Work out the finished part from the listing and answer in its coordinate system (mm). A direction names the side the tool comes from. Round coordinates to 2 decimals unless told otherwise and drop trailing zeros. Order: outer loops, then holes, each group sorted by start corner. A loop starts at its lowest first (then second) coordinate and runs counter-clockwise, first axis right, second up. Notation, with made-up numbers: M 54,-30 L 67,-30 A12 cw 67,-17 Z; hole C 71.5,4.5 d5. An arc over 180 degrees is marked long. Answer as a JSON object with one key per item and string values. Group by question number.
from build123d import *

# Parameters (mm, degrees)
F0_W     = 406.4
F0_H     = 304.8
F1_DEPTH = 2.54
F2_W     = 7.62
F2_H     = 7.62
F3_DEPTH = 88.9
F4_W     = 203.2
F4_H     = 203.2
F5_DEPTH = 165.1
F7_DEPTH = 203.2
F8_W     = 7.62
F8_H     = 297.18
F9_DEPTH = 7.62


with BuildPart() as f1:
    # F0 (on Top) → F1 (new body)
    with BuildSketch(Plane.XY):
        with Locations((-190.104838, 115.129152)):
            Rectangle(F0_W, F0_H)
    extrude(amount=F1_DEPTH)

    # F2 (on face) → F3 (join)
    with BuildSketch(Plane.XY.offset(2.54)):
        with Locations((-389.494838, -33.460848)):
            Rectangle(F2_W, F2_H)
        with Locations((9.285162, -33.460848)):
            Rectangle(F2_W, F2_H)
        with Locations((9.285162, 263.719152)):
            Rectangle(F2_W, F2_H)
    extrude(amount=F3_DEPTH)

    # F4 (on face) → F5 (join)
    with BuildSketch(Plane.XY.offset(2.54)):
        with Locations((-291.704838, 165.929152)):
            Rectangle(F4_W, F4_H)
    extrude(amount=F5_DEPTH)

    # F6 (on face) → F7 (join)
    with BuildSketch(Plane.XZ.offset(-64.329152)):
        Polygon((-291.704838, 231.14), (-393.304838, 167.64), (-291.704838, 167.64), align=None)
        Polygon((-291.704838, 231.14), (-291.704838, 167.64), (-190.104838, 167.64), align=None)
    extrude(amount=-F7_DEPTH)

    # F8 (on face) → F9 (join)
    with BuildSketch(Plane.XY.offset(91.44)):
        Polygon((-393.304838, -37.270848), (13.095162, -37.270848), (13.095162, -29.650848), (5.475162, -29.650848), (-393.304838, -29.650848), align=None)
        with Locations((9.285162, 118.939152)):
            Rectangle(F8_W, F8_H)
    extrude(amount=F9_DEPTH)


solid = f1.part
Item 1: Find section C-C (z = 83.5). Give the vertices of the cut face in (x, y).
Item 2: Find section D-D (y = 8). Give the vertices of the cut face in (x, z).
Item 3: Consider L1, parallel to X at y = 93.5, z = 92.5; L2, parallel to Y at x = -272, z = 96; L3, parallel to X at y = 130, z = 14. Determine where each line is inside the solid, lowest interval first.
Item 4: The mould has two halves that part along Y. Classify faces 4 (the flat face through (-341.794, 164.507, 199.834)), 5 (the flat face through (-251, -37.271, 93)), 6 (the flat face through (-283, 267.529, 88)), 7 (the flat face through (-193, -29.651, 93)): +Y half, -Y half, draft (parallel to the pull), parting line (faces both ways), or undercut.
Item 5: Each of these flat-tipped pins is pushed along its axis until it touches: pin 1 (5 mm diameter, centred on y = 143, z = 169, fed in from +X); pin 2 (4 mm diameter, centred on x = -323.5, z = 106.5, fed in from -Y); pin 3 (3 mm diameter, centred on x = -216, y = 4, fed in from +Z). Where does it stop, or does it pass through?
Item 6: Find section B-B (x = -99). Give the vertices of the cut face in (y, z).
Item 7: Find section A-A (y = 200.5). Give the vertices of the cut face in (x, z), and give its area (3 significant figures).
Item 8: A tool of negligible diameter and unlimited length cuts with its end or side. For faces 1 (the flat face through (-293, 64.329, 93)), 2 (the flat face through (-193, 117, 0)), 3 (the flat face through (5.475, 162, 93)), from which of +Z, -Z, +X, -X, +Y, -Y can it reach the whole face along a straight path? Write none if from no direction.
Responses:
{
 "1": {"outline": "M -393.3,-37.27 L -385.68,-37.27 L -385.68,-29.65 L -393.3,-29.65 Z; M -393.3,64.33 L -190.1,64.33 L -190.1,267.53 L -393.3,267.53 Z; M 5.48,-37.27 L 13.1,-37.27 L 13.1,-29.65 L 5.48,-29.65 Z; M 5.48,259.91 L 13.1,259.91 L 13.1,267.53 L 5.48,267.53 Z"},
 "2": {"outline": "M -393.3,0 L 13.1,0 L 13.1,2.54 L -393.3,2.54 Z; M 5.48,91.44 L 13.1,91.44 L 13.1,99.06 L 5.48,99.06 Z"},
 "3": {"L1": "x = -393.3 to -190.1, 5.48 to 13.1", "L2": "y = -37.27 to -29.65, 64.33 to 267.53", "L3": "x = -393.3 to -190.1"},
 "4": {"face 4": "draft", "face 5": "-Y half", "face 6": "+Y half", "face 7": "undercut"},
 "5": {"pin 1": "stops at x = -190.1", "pin 2": "stops at y = 64.33", "pin 3": "stops at z = 2.54"},
 "6": {"outline": "M -37.27,0 L 267.53,0 L 267.53,2.54 L -37.27,2.54 Z; M -37.27,91.44 L -29.65,91.44 L -29.65,99.06 L -37.27,99.06 Z"},
 "7": {"outline": "M -393.3,0 L 13.1,0 L 13.1,2.54 L -190.1,2.54 L -190.1,167.64 L -291.7,231.14 L -393.3,167.64 Z; M 5.48,91.44 L 13.1,91.44 L 13.1,99.06 L 5.48,99.06 Z", "area": "41,100 mm^2"},
 "8": {"face 1": "+Z, -X", "face 2": "-Z, +X, -X, +Y, -Y", "face 3": "+Z, +Y"}
}
